```python
from build123d import *

# Parameters (mm, degrees)
EXTRUDE_1_DEPTH     = 440
CUT_EXTRUDE_1_DEPTH = 30.906162578


with BuildPart() as part:
    # Эскиз1 → Бобышка-Вытянуть1 (new body)
    with BuildSketch(Plane.XY):
        Polygon((169.252902227, 0), (0, 0), (0, -1), (16.565023393, -15), (144.748239349, -15), (144.748239349, -16), (152.776966057, -29.906162578), (170.193520621, -29.906162578), align=None)
    extrude(amount=-EXTRUDE_1_DEPTH)

    # Эскиз4 → Вырез-Вытянуть1 (cut, through all)
    with BuildSketch(Plane(origin=(0, 0, 0), x_dir=(1, 0, 0), z_dir=(0, 1, 0))):
        with BuildLine():
            Line((75.748239349, 65), (75.748239349, 45))
            ThreePointArc((75.748239349, 45), (94.748239349, 26), (113.748239349, 45))
            Line((113.748239349, 45), (113.748239349, 65))
            ThreePointArc((113.748239349, 65), (94.748239349, 84), (75.748239349, 65))
        make_face()
        with BuildLine():
            Line((75.748239349, 395), (75.748239349, 375))
            ThreePointArc((75.748239349, 375), (94.748239349, 356), (113.748239349, 375))
            Line((113.748239349, 375), (113.748239349, 395))
            ThreePointArc((113.748239349, 395), (94.748239349, 414), (75.748239349, 395))
        make_face()
    extrude(amount=-CUT_EXTRUDE_1_DEPTH, mode=Mode.SUBTRACT)


solid = part.part
```
Input: part model. Units: mm. Frame: model coordinates. A direction names the side the tool comes from. Round coordinates to 2 decimals unless told otherwise and drop trailing zeros. Order: outer loops, then holes, each group sorted by start corner. A loop starts at its lowest first (then second) coordinate and runs counter-clockwise, first axis right, second up. Notation, with made-up numbers: (-24.75, 9.25) - (12.25, 9.25) arc R21 cw to (12.25, 23.25) - close; hole circle Ø1 at (28, -34.75). An arc over 180 degrees is marked (long way). One line per question, with ' | ' between items. Start each with the question number.
1) Pull-direction query (X, two-part tool) for faces 4 (the flat face through (148.71, -22.86, -216.92)), 5 (the flat face through (113.748, -7, -55)), 6 (the flat face through (161, -29.906, -217)); classes: +X half, -X half, draft (parallel to the pull), parting line (faces both ways), or undercut.
2) Contact query for flat-ended pins moving along their axis: P1, Ø8, axis at y = -17.5, z = -236, coming from the -X side; P2, Ø5, axis at y = -25.5, z = -355, coming from the -X side; P3, Ø5, axis at x = 85, z = -224, coming from the -Y side. Output: stop coordinate, or through.
3) Cut plane C-C, the plane y = -22. Return the cut outline in (x, z).
4) Ray query, probe 1 along Y at (x, z) = (103.5, -126); probe 2 along X at (y, z) = (-3.5, -412); probe 3 along X at (y, z) = (-1.75, -261.5). Return the intervals inside material, ascending.
5) Set-up query: faces 1 (the flat face through (103, -8, 0)), 2 (the flat face through (80, -15, -217)), 3 (the cylindrical face through (94.33, -7.395, -26.005)). Return all of +Z, -Z, +X, -X, +Y, -Y with unobstructed straight access to the full face (end or side cutting, diameter ignored); none if empty.
6) Cut plane A-A, the plane z = -329. Return the cut outline in (x, y).
7) Cut plane B-B, the plane x = 120.5. Return the cut outline in (y, z), then the cut area to 3 significant figures.
Worked out:
1) face 4: -X half | face 5: undercut | face 6: draft
2) P1: stops at x = 14.79 | P2: stops at x = 148.79 | P3: stops at y = -15
3) outline: (148.21, -440) - (169.94, -440) - (169.94, 0) - (148.21, 0) - close
4) probe 1: y = -15 to 0 | probe 2: x = 2.96 to 86.26, 103.23 to 169.36 | probe 3: x = 0.89 to 169.31
5) face 1: +Z, +X, -X, +Y, -Y | face 2: +Z, -Z, -X, -Y | face 3: +Y, -Y
6) outline: (0, -1) - (16.57, -15) - (144.75, -15) - (144.75, -16) - (152.78, -29.91) - (170.19, -29.91) - (169.25, 0) - (0, 0) - close
7) outline: (-15, -440) - (0, -440) - (0, 0) - (-15, 0) - close | area: 6,600 mm^2
